Geometry check sheet. Reference: the model listing, model coordinates, mm. A direction names the side the tool comes from. Coordinates: 2 decimals unless noted, no trailing zeros. Order: outer loops, then holes, each group sorted by start corner. A loop starts at its lowest first (then second) coordinate and runs counter-clockwise, first axis right, second up.
```python
from build123d import *
from build123d.topology import SkipClean

# Parameters (mm, degrees)
CROQUIS1_R              = 14.5
SALIENTE_EXTRUIR1_DEPTH = 35
CROQUIS2_R              = 2.4
SALIENTE_EXTRUIR2_DEPTH = 43
SALIENTE_EXTRUIR3_DEPTH = 14.5
SALIENTE_EXTRUIR4_START = 6
CROQUIS4_R              = 2.4
SALIENTE_EXTRUIR4_DEPTH = 6


with BuildPart() as part:
    # Croquis1 → Saliente-Extruir1 (new, symmetric)
    with BuildSketch(Plane(origin=(0, 0, 0), x_dir=(1, 0, 0), z_dir=(0, 1, 0))):
        with Locations(Location((0, 0, 0), (0, 0, 270))):
            Circle(CROQUIS1_R)
    extrude(amount=SALIENTE_EXTRUIR1_DEPTH, both=True)

    # Croquis2 → Saliente-Extruir2 (add, symmetric)
    with BuildSketch(Plane(origin=(0, 0, 0), x_dir=(1, 0, 0), z_dir=(0, 1, 0))):
        with Locations(Location((0, 0, 0), (0, 0, 270))):
            Circle(CROQUIS2_R)
    extrude(amount=SALIENTE_EXTRUIR2_DEPTH, both=True)

    # Croquis3 → Saliente-Extruir3 (add)
    with SkipClean():  # the faces are left unmerged after this step: merging them gives an invalid solid
        with BuildSketch(Plane.XZ.offset(43)):
            with BuildLine():
                Line((-1.75, 1.642406771), (-1.75, -1.642406771))
                ThreePointArc((-1.75, -1.642406771), (0, -2.4), (1.75, -1.642406771))
                Line((1.75, -1.642406771), (1.75, 1.642406771))
                ThreePointArc((1.75, 1.642406771), (0, 2.4), (-1.75, 1.642406771))
            make_face()
        extrude(amount=SALIENTE_EXTRUIR3_DEPTH)

    # Croquis4 → Saliente-Extruir4 (add)
    with SkipClean():  # the faces are left unmerged after this step: merging them gives an invalid solid
        with BuildSketch(Plane(origin=(0, 43, 0), x_dir=(1, 0, 0), z_dir=(0, 1, 0)).offset(SALIENTE_EXTRUIR4_START)):
            with Locations(Location((0, 0, 0), (0, 0, 43.183421796))):
                Circle(CROQUIS4_R)
        extrude(amount=-SALIENTE_EXTRUIR4_DEPTH)


solid = part.part
```
Item 1: Sectioned sample at D-D (z = 9.5). Record the cut outline in (x, y), and give its area (3 significant figures).
Item 2: Thickness scan on line 1 along Y through (x, z) = (-12.5, -2.25); line 2 along X through (y, z) = (-32, 0.5); line 3 along X through (y, z) = (-50.5, -0.75). Record the ranges inside material, lowest first.
Item 3: Tool access check on faces 1 (the face through (1.75, -50, 0)), 2 (the face through (0, 49, 0)), 3 (the face through (-1.75, -50, 0)). Record the directions out of +Z, -Z, +X, -X, +Y, -Y that give a thin tool (end or side, any length) a straight path to the whole face; none if there is none.
Item 4: Sectioned sample at A-A (z = 0). Record the cut outline in (x, y), and give its area (3 significant figures).
Item 5: Sectioned sample at B-B (y = 33). Record the cut outline in (x, z), and give its area (3 significant figures).
Item 6: Sectioned sample at C-C (z = -12). Record the cut outline in (x, y).
Item 7: Depth check by flat-ended pin: P1, Ø3, axis at y = -19.5, z = 7.5, coming from the +X side; P2, Ø3, axis at x = 9, y = 32, coming from the -Z side; P3, Ø1.5, axis at y = -24, z = 11, coming from the +X side; P4, Ø0.7, axis at x = 2, z = 0, coming from the -Y side. Enter the tip coordinate at first touch or a pass-through.
Geometry check:
1. outline: (-10.95, -35) - (10.95, -35) - (10.95, 35) - (-10.95, 35) - close
1. area: 1,530 mm2
2. line 1: y = -35 to 35
2. line 2: x = -14.49 to 14.49
2. line 3: x = -1.75 to 1.75
3. face 1: +Z, -Z, +X, -Y
3. face 2: +Z, -Z, +X, -X, +Y
3. face 3: +Z, -Z, -X, -Y
4. outline: (-14.5, -35) - (-2.4, -35) - (-2.4, -43) - (-1.75, -43) - (-1.75, -57.5) - (1.75, -57.5) - (1.75, -43) - (2.4, -43) - (2.4, -35) - (14.5, -35) - (14.5, 35) - (2.4, 35) - (2.4, 49) - (-2.4, 49) - (-2.4, 35) - (-14.5, 35) - close
4. area: 2,190 mm2
5. outline: circle Ø29 at (0, 0)
5. area: 661 mm2
6. outline: (-8.14, -35) - (8.14, -35) - (8.14, 35) - (-8.14, 35) - close
7. P1: stops at x = 13.2
7. P2: stops at z = -12.41
7. P3: stops at x = 10.26
7. P4: stops at y = -57.5
